The listing builds one solid part. Answer for the finished solid, in the listing's coordinates (mm). A direction names the side the tool comes from. Coordinates: 2 decimals unless noted, no trailing zeros. Loops run counter-clockwise (first coordinate to the right, second up) from the corner with the lowest first, then second, coordinate; pieces in that order, holes last. Notation, with made-up numbers: M 2.25,87 L 33.25,87 A25 ccw 33.25,125 Z; hole C -33,69 d11. An arc over 180 degrees is marked long. Return JSON: item names as keys, results as strings. Group by question number.
1. Section D-D (x = -58) is taken. Write down the section's boundary in (y, z).
2. The mould has two halves that part along Z. Classify faces 1 (the face through (6.072, 7.703, -63.636)), 2 (the face through (63.4, 7.7, -8.2)), 3 (the face through (16, 4.572, -1)): pulls with the +Z half, pulls with the -Z half, needs draft (parallel to the pull), parting line crosses it, or undercut.
3. Given P1, Ø3, axis at y = 4, z = -11.5, coming from the +X side; P2, Ø6, axis at y = 10, z = -19, coming from the +X side; P3, Ø1, axis at x = -56, y = 8.5, coming from the +Z side, each flat-ended and moving along its own axis, determine where each tip first touches the part or whether it passes through.
4. Which of the six approach directions +Z, -Z, +X, -X, +Y, -Y give full straight-line access (tool end or side, diameter ignored) to faces 4 (the face through (-5.023, 2.254, -6.551)), 5 (the face through (60.69, 7.7, 20.08))?
5. Section C-C (z = 0) is taken. Write down the section's boundary in (x, y) (1 decimal).
6. Section B-B (x = 0) is taken. Write down the section's boundary in (y, z) (1 decimal), then the cut area to 3 significant figures.
7. Straight lines are drawn through the part: L1, parallel to X at y = 2.9, z = 0 (1 decimal); L2, parallel to Y at x = 47, z = 29; L3, parallel to X at y = 5.75, z = 63. For each, find the intervals that lie inside material, in ascending order. Write a range as from..to.
```python
from build123d import *

# Parameters (mm, degrees)
SKETCH1_R           = 8.255
BOSS_EXTRUDE1_DEPTH = 4.572
BOSS_EXTRUDE2_DEPTH = 6.35


# Read off the part's stored shape, not the designer's step: Boss-Extrude2
with BuildPart() as part:
    # Sketch1 → Boss-Extrude1 (new body)
    with BuildSketch(Plane(origin=(0, 0, 0), x_dir=(1, 0, 0), z_dir=(0, 1, 0))):
        with Locations(Location((0, 0, 0), (0, 0, 270))):
            Circle(SKETCH1_R)
        with BuildLine():
            Line((2.236967199, -1.778), (2.236967199, 1.778))
            ThreePointArc((2.236967199, 1.778), (-2.8575, 0), (2.236967199, -1.778))
        make_face(mode=Mode.SUBTRACT)
    extrude(amount=BOSS_EXTRUDE1_DEPTH)

    # Boss-Extrude2 outline → Boss-Extrude2 (add)
    with BuildSketch(Plane(origin=(0, 4.572, 0), x_dir=(1, 0, 0), z_dir=(0, 1, 0))):
        with BuildLine():
            ThreePointArc((75.887851324, -6.890139437), (63.350649048, 8.530748581), (71.362110957, 26.718703558))
            ThreePointArc((71.362110957, 26.718703558), (53.375609462, 35.172755376), (52.702229316, 55.03557963))
            ThreePointArc((52.702229316, 55.03557963), (32.828875813, 54.848366603), (23.604024808, 72.451984189))
            ThreePointArc((23.604024808, 72.451984189), (5.779980689, 63.660586154), (-10.169246297, 75.518384714))
            ThreePointArc((-10.169246297, 75.518384714), (-22.413710496, 59.86404587), (-41.928373455, 63.627442974))
            ThreePointArc((-41.928373455, 63.627442974), (-46.168091432, 44.210697118), (-65.383072033, 39.134305814))
            ThreePointArc((-65.383072033, 39.134305814), (-60.778315646, 19.800877593), (-75.887851324, 6.890139437))
            ThreePointArc((-75.887851324, 6.890139437), (-63.350649048, -8.530748581), (-71.362110957, -26.718703558))
            ThreePointArc((-71.362110957, -26.718703558), (-53.375609462, -35.172755376), (-52.702229316, -55.03557963))
            ThreePointArc((-52.702229316, -55.03557963), (-32.828875813, -54.848366603), (-23.604024808, -72.451984189))
            ThreePointArc((-23.604024808, -72.451984189), (-5.779980689, -63.660586154), (10.169246297, -75.518384714))
            ThreePointArc((10.169246297, -75.518384714), (22.413710496, -59.86404587), (41.928373455, -63.627442974))
            ThreePointArc((41.928373455, -63.627442974), (46.168091432, -44.210697118), (65.383072033, -39.134305814))
            ThreePointArc((65.383072033, -39.134305814), (60.778315646, -19.800877593), (75.887851324, -6.890139437))
        make_face()
        with BuildLine():
            Line((2.236967199, 1.778), (2.236967199, -1.778))
            ThreePointArc((2.236967199, -1.778), (-2.8575, 0), (2.236967199, 1.778))
        make_face(mode=Mode.SUBTRACT)
    extrude(amount=BOSS_EXTRUDE2_DEPTH)


solid = part.part
```
Worked out:
{
 "1": {"outline": "M 4.57,-38.43 L 10.92,-38.43 L 10.92,30.31 L 4.57,30.31 Z"},
 "2": {"face 1": "pulls with the -Z half", "face 2": "undercut", "face 3": "needs draft"},
 "3": {"P1": "x = 63.27", "P2": "x = 66.63", "P3": "z = 32.5"},
 "4": {"face 4": "-Y", "face 5": "+X, +Y, -Y"},
 "5": {"outline": "M -66.7,4.6 L -8.3,4.6 L -8.3,0 L -2.9,0 L -2.9,10.9 L -66.7,10.9 Z; M 2.2,0 L 8.3,0 L 8.3,4.6 L 66.7,4.6 L 66.7,10.9 L 2.2,10.9 Z"},
 "6": {"outline": "M 0,-8.3 L 4.6,-8.3 L 4.6,-65.1 L 10.9,-65.1 L 10.9,-2.9 L 0,-2.9 Z; M 0,2.9 L 10.9,2.9 L 10.9,65.1 L 4.6,65.1 L 4.6,8.3 L 0,8.3 Z", "area": "840 mm^2"},
 "7": {"L1": "-8.3..-2.9, 2.2..8.3", "L2": "4.57..10.92", "L3": "-25.41..16.98, 41.2..41.72"}
}
